Autodesk Inventor part; units mm, degrees
ref_plane "YZ Plane" through (0, 0, 0) normal (1, 0, 0) x (0, 1, 0)
ref_plane "XZ Plane" through (0, 0, 0) normal (0, 1, 0) x (-1, 0, 0)
ref_plane "XY Plane" through (0, 0, 0) normal (0, 0, 1) x (1, 0, 0)
sketch "Sketch1" plane through (0, 0, 0) normal (0, 0, 1) x (1, 0, 0)
  line L0 (0, 0) -> (-47.5, 0)
  line L1 (-47.5, 0) -> (-72.2487, 24.7487)
  line L2 (-72.2487, 24.7487) -> (-72.2487, 72.2487)
  line L3 (-72.2487, 72.2487) -> (0, 72.2487)
  line L4 (0, 72.2487) -> (0, 0)
  line L5 (0, 144.4975) -> (-47.5, 144.4975)
  line L6 (-47.5, 144.4975) -> (-72.2487, 119.7487)
  line L7 (-72.2487, 119.7487) -> (-72.2487, 72.2487)
  line L8 (0, 0) -> (47.5, 0)
  line L9 (47.5, 0) -> (72.2487, 24.7487)
  line L10 (72.2487, 24.7487) -> (72.2487, 72.2487)
  line L11 (72.2487, 119.7487) -> (72.2487, 72.2487)
  line L12 (47.5, 144.4975) -> (72.2487, 119.7487)
  line L13 (0, 144.4975) -> (47.5, 144.4975)
  dimension "d0" = 47.5
  dimension "d2" = 35
  dimension "d3" = 135
extrude "Extrusion1" add sketch "Sketch1" along normal mid plane 3
sketch "Sketch2" plane through (0, 0, 1.5) normal (0, 0, 1) x (1, 0, 0)
  line L0 (-32.5, 97.5) -> (-22.5, 97.5)
  line L1 (-22.5, 97.5) -> (-22.5, 47.5)
  line L2 (-22.5, 47.5) -> (-32.5, 47.5)
  line L3 (-32.5, 47.5) -> (-32.5, 97.5)
  line L4 (0, 0) -> (0, 144.4975)
  line L5 (-47.5, 144.4975) -> (47.5, 144.4975)
  line L6 (-47.5, 0) -> (47.5, 0)
  line L7 (32.5, 97.5) -> (22.5, 97.5)
  line L8 (22.5, 97.5) -> (22.5, 47.5)
  line L9 (22.5, 47.5) -> (32.5, 47.5)
  line L10 (32.5, 47.5) -> (32.5, 97.5)
  dimension "d6" = 50
  dimension "d7" = 10
  dimension "d8" = 45
  dimension "d10" = 47.5
extrude "Extrusion2" cut sketch "Sketch2" against normal blind 3
sketch "Sketch3" plane through (0, 0, 1.5) normal (0, 0, 1) x (1, 0, 0)
  line L0 (47.5, 144.4975) -> (-47.5, 144.4975)
  line L1 (0, 144.4975) -> (0, 0)
  line L2 (-72.2487, 119.7487) -> (-72.2487, 24.7487)
  line L3 (-72.2487, 72.2487) -> (0, 72.2487)
  circle A0 centre (-57.3995, 14.8492) radius 1.25
  line L4 (-72.2487, 24.7487) -> (-47.5, 0)
  line L5 (-59.8744, 12.3744) -> (0, 72.2487)
  circle A1 centre (-57.3995, 129.6482) radius 1.25
  circle A2 centre (57.3995, 14.8492) radius 1.25
  circle A3 centre (57.3995, 129.6482) radius 1.25
  dimension "d13" = 2.5
  dimension "d14" = 3.5
extrude "Extrusion3" add sketch "Sketch3" along normal blind 0.1 contours L5 A0 | A0 L5 | A1 | A2 | A3
properties part number "Middle_base"
Input: part model. Units: mm. Frame: model coordinates. Coordinates: 2 decimals unless noted, no trailing zeros. Loops run counter-clockwise (first coordinate to the right, second up) from the corner with the lowest first, then second, coordinate; pieces in that order, holes last. Notation, with made-up numbers: (61, -4.75) -> (93, -4.75) arc R22 cw to (93, 24.25) -> close; hole circle Ø10 at (0, 48). An arc over 180 degrees is marked (long way). One line per item, written item: value.
(1) Cut plane B-B (x = -27.5). Output: boundary loops of the cut face in (y, z), then the cut area to 3 significant figures.
Answer below:
outline: (0, -1.5) -> (47.5, -1.5) -> (47.5, 1.5) -> (0, 1.5) -> close; (97.5, -1.5) -> (144.5, -1.5) -> (144.5, 1.5) -> (97.5, 1.5) -> close
area: 283 mm2
(2) Cut plane C-C (y = 51). Output: boundary loops of the cut face in (x, z).
Answer below:
outline: (-72.25, -1.5) -> (-32.5, -1.5) -> (-32.5, 1.5) -> (-72.25, 1.5) -> close; (-22.5, -1.5) -> (22.5, -1.5) -> (22.5, 1.5) -> (-22.5, 1.5) -> close; (32.5, -1.5) -> (72.25, -1.5) -> (72.25, 1.5) -> (32.5, 1.5) -> close
(3) Ray query, line 1 along X through (y, z) = (79.5, -0.05); line 2 along Y through (x, z) = (-28, 0.35); line 3 along Z through (x, y) = (-27.5, 132.5). Return the intervals inside material, ascending.
Answer below:
line 1: x = -72.25 to -32.5, -22.5 to 22.5, 32.5 to 72.25
line 2: y = 0 to 47.5, 97.5 to 144.5
line 3: z = -1.5 to 1.5
(4) Cut plane D-D (y = 100). Output: boundary loops of the cut face in (x, z).
Answer below:
outline: (-72.25, -1.5) -> (72.25, -1.5) -> (72.25, 1.5) -> (-72.25, 1.5) -> close
(5) Cut plane A-A (z = 0.85). Output: boundary loops of the cut face in (x, y).
Answer below:
outline: (-72.25, 24.75) -> (-47.5, 0) -> (47.5, 0) -> (72.25, 24.75) -> (72.25, 119.75) -> (47.5, 144.5) -> (-47.5, 144.5) -> (-72.25, 119.75) -> close; hole (-32.5, 47.5) -> (-22.5, 47.5) -> (-22.5, 97.5) -> (-32.5, 97.5) -> close; hole (22.5, 47.5) -> (32.5, 47.5) -> (32.5, 97.5) -> (22.5, 97.5) -> close
